Geometry check sheet. Reference: drawing and pictorial views, mm from the part's lowest x, y, z. Coordinates: 2 decimals unless noted, no trailing zeros. Loops run counter-clockwise (first coordinate to the right, second up) from the corner with the lowest first, then second, coordinate; pieces in that order, holes last. Notation, with made-up numbers: (9, -37.75) -> (45, -37.75) arc R19 cw to (45, -16.75) -> close; hole circle Ø4 at (-31, 20.25). An arc over 180 degrees is marked (long way). Answer as a JSON object with one key per item and string values.
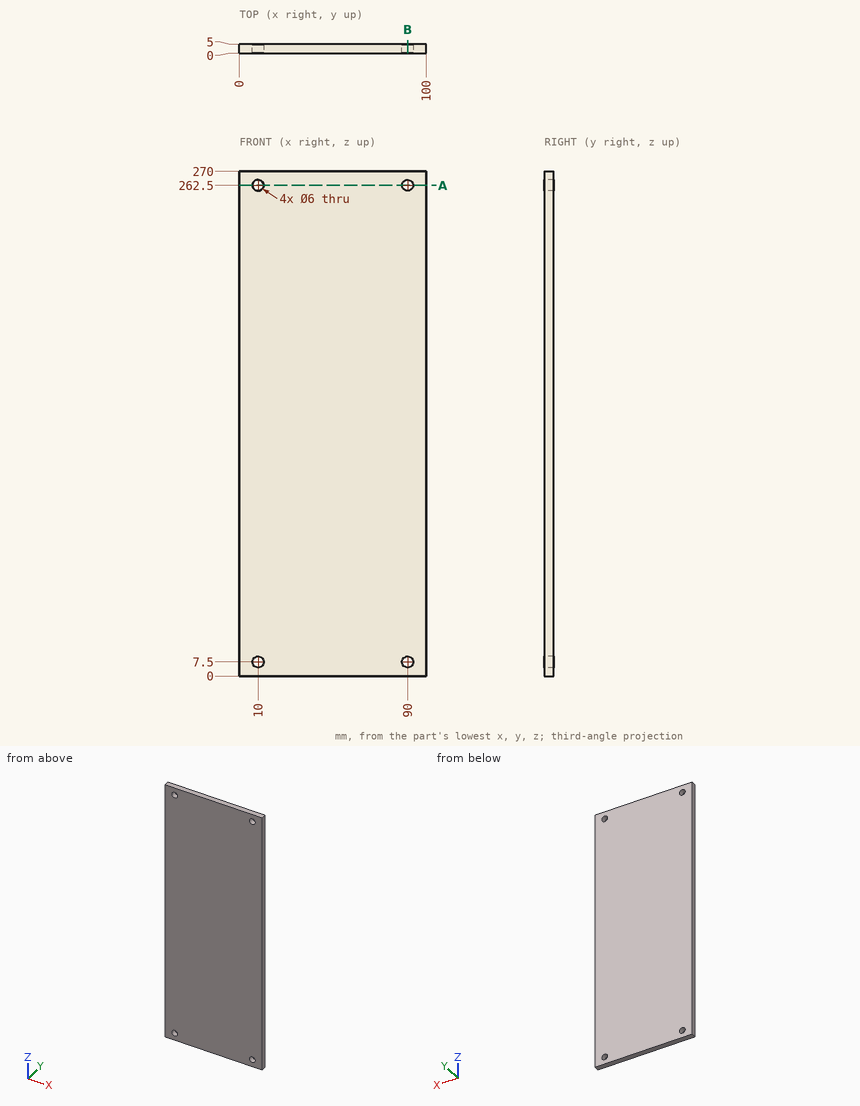
1. Thickness scan on probe 1 along X at (y, z) = (1.4, 262.5); probe 2 along Z at (x, y) = (10, 2.5); probe 3 along Z at (x, y) = (92.5, 1.65). Record the ranges inside material, lowest first. Write a range as from..to.
Evaluation:
{"probe 1": "x = 0..7, 13..87, 93..100", "probe 2": "z = 0..4.5, 10.5..259.5, 265.5..270", "probe 3": "z = 0..5.84, 9.16..260.84, 264.16..270"}
2. Section check B-B, the plane x = 90. Record the boundary of the cut face in (y, z), then the cut area to 3 significant figures.
Evaluation:
{"outline": "(0, 0) -> (5, 0) -> (5, 4.5) -> (0, 4.5) -> close; (0, 10.5) -> (5, 10.5) -> (5, 259.5) -> (0, 259.5) -> close; (0, 265.5) -> (5, 265.5) -> (5, 270) -> (0, 270) -> close", "area": "1,290 mm^2"}
3. Section check A-A, the plane z = 262.5. Record the boundary of the cut face in (x, y), then the cut area to 3 significant figures.
Evaluation:
{"outline": "(0, 0) -> (7, 0) -> (7, 5) -> (0, 5) -> close; (13, 0) -> (87, 0) -> (87, 5) -> (13, 5) -> close; (93, 0) -> (100, 0) -> (100, 5) -> (93, 5) -> close", "area": "440 mm^2"}
